from build123d import *

# Parameters (mm, degrees)
BOSS_EXTRUDE1_DEPTH = 14
CUT_EXTRUDE1_DEPTH  = 28
CUT_EXTRUDE2_DEPTH  = 28
CUT_EXTRUDE3_DEPTH  = 28
SKETCH5_R           = 5.5
CUT_EXTRUDE4_DEPTH  = 28


with BuildPart() as part:
    # Sketch1 → Boss-Extrude1 (new, symmetric)
    with BuildSketch(Plane.XY):
        Polygon((-600, 0), (600, 0), (200, -300), (-200, -300), align=None)
    extrude(amount=BOSS_EXTRUDE1_DEPTH, both=True)

    # Sketch2 → Cut-Extrude1 (cut)
    with BuildSketch(Plane.XY.offset(14)):
        Polygon((-175, -275), (175, -275), (175, -25), align=None)
        Polygon((-175, -25), (-175, -250), (150, -25), align=None)
    extrude(amount=-CUT_EXTRUDE1_DEPTH, mode=Mode.SUBTRACT)

    # Sketch3 → Cut-Extrude2 (cut)
    with BuildSketch(Plane.XY.offset(14)):
        Polygon((-525, -25), (-200, -25), (-200, -268.75), align=None)
    extrude(amount=-CUT_EXTRUDE2_DEPTH, mode=Mode.SUBTRACT)

    # Sketch4 → Cut-Extrude3 (cut)
    with BuildSketch(Plane.XY.offset(14)):
        Polygon((200, -25), (525, -25), (200, -268.75), align=None)
    extrude(amount=-CUT_EXTRUDE3_DEPTH, mode=Mode.SUBTRACT)

    # Sketch5 → Cut-Extrude4 (cut)
    with BuildSketch(Plane.XY.offset(14)):
        with Locations((-187.5, -12.5)):
            Circle(SKETCH5_R)
        with Locations((-187.5, -287.5)):
            Circle(SKETCH5_R)
        with Locations((187.5, -287.5)):
            Circle(SKETCH5_R)
        with Locations((187.5, -12.5)):
            Circle(SKETCH5_R)
        with Locations((544.11011126, -12.5)):
            Circle(SKETCH5_R)
    extrude(amount=-CUT_EXTRUDE4_DEPTH, mode=Mode.SUBTRACT)


solid = part.part
Can you work these out from the model? Positions are in its coordinate system, mm. A direction names the side the tool comes from. Give positions to 0.01 mm unless a question says otherwise; leave off trailing zeros. Loops run counter-clockwise (first coordinate to the right, second up) from the corner with the lowest first, then second, coordinate; pieces in that order, holes last. Notation, with made-up numbers: (54.25, 79.25) - (112.25, 79.25) arc R29 ccw to (112.25, 114.25) - close; hole circle Ø7 at (34, 68). An arc over 180 degrees is marked (long way). One line per item, written item: value.
(1) I need wall thicknesses on line 1 along Y through (x, z) = (187.5, -1.5); line 2 along X through (y, z) = (-49.5, 10.5); line 3 along X through (y, z) = (-287.5, -3.25). Which ranges of each line are inside material? Lowest first, please.
Verdict:
line 1: -300 to -293, -282 to -18, -7 to 0
line 2: -534 to -492.33, -200 to -175, 114.61 to 140.7, 175 to 200, 492.33 to 534
line 3: -216.67 to -193, -182 to 182, 193 to 216.67
(2) If we section it at A-A, the plane y = -181: List the corners of the cut face in (x, z) for me, plus the area to 3 significant figures.
Verdict:
outline: (-358.67, -14) - (-317, -14) - (-317, 14) - (-358.67, 14) - close; (-200, -14) - (-175, -14) - (-175, 14) - (-200, 14) - close; (-75.33, -14) - (-43.4, -14) - (-43.4, 14) - (-75.33, 14) - close; (175, -14) - (200, -14) - (200, 14) - (175, 14) - close; (317, -14) - (358.67, -14) - (358.67, 14) - (317, 14) - close
area: 4,630 mm^2
(3) If we mould it in two halves opening along Y, with no side actions, what happens to faces 3 (the face through (3, -138, -14)), 4 (the face through (-2, -275, 0)), 5 (the face through (402.8, -147.9, 0.2))? For each: released by +Y, released by -Y, zero draft, split by the parting line, or undercut.
Verdict:
face 3: zero draft
face 4: undercut
face 5: released by -Y
(4) If we section it at D-D, the plane x = -134: List the corners of the cut face in (y, z) for me.
Verdict:
outline: (-300, -14) - (-275, -14) - (-275, 14) - (-300, 14) - close; (-245.71, -14) - (-221.62, -14) - (-221.62, 14) - (-245.71, 14) - close; (-25, -14) - (0, -14) - (0, 14) - (-25, 14) - close
(5) If we section it at C-C, the plane z = -1.75: State how many separate pieces and enclosed holes the cut face has, plus the area to 3 significant figures.
Verdict:
separate pieces: 1
enclosed holes: 9
area: 80,000 mm^2
(6) If we section it at B-B, the plane x = 427.5: List the corners of the cut face in (y, z) for me (3 decimals), plus the area to 4 significant figures.
Verdict:
outline: (-129.375, -14) - (-98.125, -14) - (-98.125, 14) - (-129.375, 14) - close; (-25, -14) - (0, -14) - (0, 14) - (-25, 14) - close
area: 1,575 mm^2
(7) I'm going to push flat-ended pins straight in: pin 1 (8.5 mm diameter, centred on y = -182, z = 0, fed in from +X); pin 2 (10 mm diameter, centred on x = 339.5, z = -0.5, fed in from -Y) (3 decimals); pin 3 (2 mm diameter, centred on y = -32, z = 3, fed in from +X). Where does each tip first touch, or does it pass through?
Verdict:
pin 1: x = 363
pin 2: y = -199.125
pin 3: x = 558.67
(8) On a 3-axis mill with a long thin cutter (end or side, diameter ignored), from which of +Z, -Z, +X, -X, +Y, -Y can I reach the whole of each face in a straight line? I mean faces 1 (the face through (-10, -25, 0)), 2 (the face through (-8, 0, 0)). Say none if no direction works.
Verdict:
face 1: +Z, -Z
face 2: +Z, -Z, +X, -X, +Y
